Input: part model. Units: mm. Frame: model coordinates. A direction names the side the tool comes from. Give positions to 0.01 mm unless a question says otherwise; leave off trailing zeros. Write each loop counter-clockwise with the first axis right and the second up, starting at its lowest first coordinate (ties: lowest second). Pieces come first, ordered by that corner, then holes.
Autodesk Inventor part; units mm, degrees
ref_plane "YZ Plane" through (0, 0, 0) normal (1, 0, 0) x (0, 1, 0)
ref_plane "XZ Plane" through (0, 0, 0) normal (0, 1, 0) x (-1, 0, 0)
ref_plane "XY Plane" through (0, 0, 0) normal (0, 0, 1) x (1, 0, 0)
sketch "Sketch1" plane through (0, 0, 0) normal (0, 1, 0) x (-1, 0, 0)
  line L0 (0, 0) -> (25, 0)
  line L1 (25, 0) -> (25, -25)
  line L2 (25, -25) -> (0, -25)
  line L3 (0, -25) -> (0, 0)
  line L4 (22, -22) -> (22, -3)
  line L5 (22, -3) -> (3, -3)
  line L6 (3, -3) -> (3, -22)
  line L7 (3, -22) -> (22, -22)
  dimension "d0" = 25
  dimension "d1" = 25
  dimension "d2" = 3
extrude "Extrusion1" add sketch "Sketch1" along normal blind 55
sketch "Sketch2" plane through (0, 0, 0) normal (1, 0, 0) x (0, 0, -1)
  line L0 (0, 0) -> (25, 0)
  line L1 (25, 0) -> (25, 55)
  line L2 (0, 55) -> (25, 55)
  line L3 (0, 0) -> (0, 55)
  line L4 (25, 0) -> (25, 55)
  line L5 (25, 0) -> (0, 25)
  line L6 (0, 0) -> (0, 55)
  dimension "d5" = 45
extrude "Extrusion2" cut sketch "Sketch2" against normal blind 55 contours L3 L5 L0
properties part number "P410" material "Aluminum 6061"
Item 1: Ray query, line 1 (X direction, y = 18.5, z = -16); line 2 (Z direction, x = -20, y = 8.5). Return the intervals inside material, ascending.
Item 2: Section B-B (y = 37.5). Return loops of the section in (x, z), and give its area (3 significant figures).
Item 3: Set-up query: faces 4 (the flat face through (-25, 33, -12)), 5 (the flat face through (-12, 29, -22)). Return all of +Z, -Z, +X, -X, +Y, -Y with unobstructed straight access to the full face (end or side cutting, diameter ignored); none if empty.
Item 4: Section D-D (y = 12.5). Return loops of the section in (x, z).
Item 5: Mould query, pull axis Z, two halves, no side actions, for faces 1 (the flat face through (-13, 38, -3)), 2 (the flat face through (-12, 40, 0)), 3 (the flat face through (0, 33, -13)). Classes: +Z half, -Z half, draft (parallel to the pull), parting line (faces both ways), or undercut.
Item 6: Section A-A (z = -20.75). Return loops of the section in (x, y).
Item 7: Section C-C (x = -4). Return loops of the section in (y, z).
Solved:
1. line 1: x = -25 to -22, -3 to 0
1. line 2: z = -25 to -22
2. outline: (-25, -25) - (0, -25) - (0, 0) - (-25, 0) - close; hole (-22, -22) - (-3, -22) - (-3, -3) - (-22, -3) - close
2. area: 264 mm2
3. face 4: +Z, -Z, -X, +Y, -Y
3. face 5: +Y, -Y
4. outline: (-25, -25) - (0, -25) - (0, -12.5) - (-3, -12.5) - (-3, -22) - (-22, -22) - (-22, -12.5) - (-25, -12.5) - close
5. face 1: undercut
5. face 2: +Z half
5. face 3: draft
6. outline: (-25, 4.25) - (-22, 4.25) - (-22, 55) - (-25, 55) - close; (-3, 4.25) - (0, 4.25) - (0, 55) - (-3, 55) - close
7. outline: (0, -25) - (55, -25) - (55, -22) - (3, -22) - close; (22, -3) - (55, -3) - (55, 0) - (25, 0) - close
